Design review of the part shown in the three views and the two pictorial views. Dimensions are in mm from the part's minimum x, y and z. A direction names the side the tool comes from. Give positions to 0.01 mm unless a question says otherwise; leave off trailing zeros. Loops run counter-clockwise (first coordinate to the right, second up) from the corner with the lowest first, then second, coordinate; pieces in that order, holes last. Notation, with made-up numbers: (29, 73) -> (75, 73) arc R17 ccw to (75, 93) -> close; hole circle Ø8 at (4.5, -15). An arc over 180 degrees is marked (long way). Use CSV: the item, a comma, the result in double quotes. Start each with the question number.
Item 1: Clearance check with flat-ended pins moving along their axes: pin 1 (1.6 mm diameter, centred on x = 29.5, y = 1, fed in from -Z); pin 2 (2.5 mm diameter, centred on x = 2.5, z = 33.5, fed in from -Y); pin 3 (1.8 mm diameter, centred on x = 19.5, z = 1.5, fed in from +Y); pin 4 (4 mm diameter, centred on y = 7.5, z = 6.5, fed in from -X). State where each tip first meets the part, or that it passes through.
Item 2: We need section A-A (x = 2.5). State the section outline as (y, z) points.
Item 3: We need section B-B (z = 33.5). State the section outline as (x, y) points.
Item 4: We need section C-C (x = 44.5). State the section outline as (y, z) points.
Item 5: For the marked faces 1, 2 and 3, list the 3-axis set-ups (+Z, -Z, +X, -X, +Y, -Y) from which the entire face can be reached by the end or side of a thin tool; tool diameter is ignored.
Item 6: Wall thickness on line 1 along X through (y, z) = (2.55, 2.5); line 2 along Z through (x, y) = (77.5, 3.1); line 3 along Z through (x, y) = (19, 4.25): over which ranges is each line inside the solid? List them lowest first. Write a range as from..to.
Item 7: We need section D-D (z = 9). State the section outline as (x, y) points.
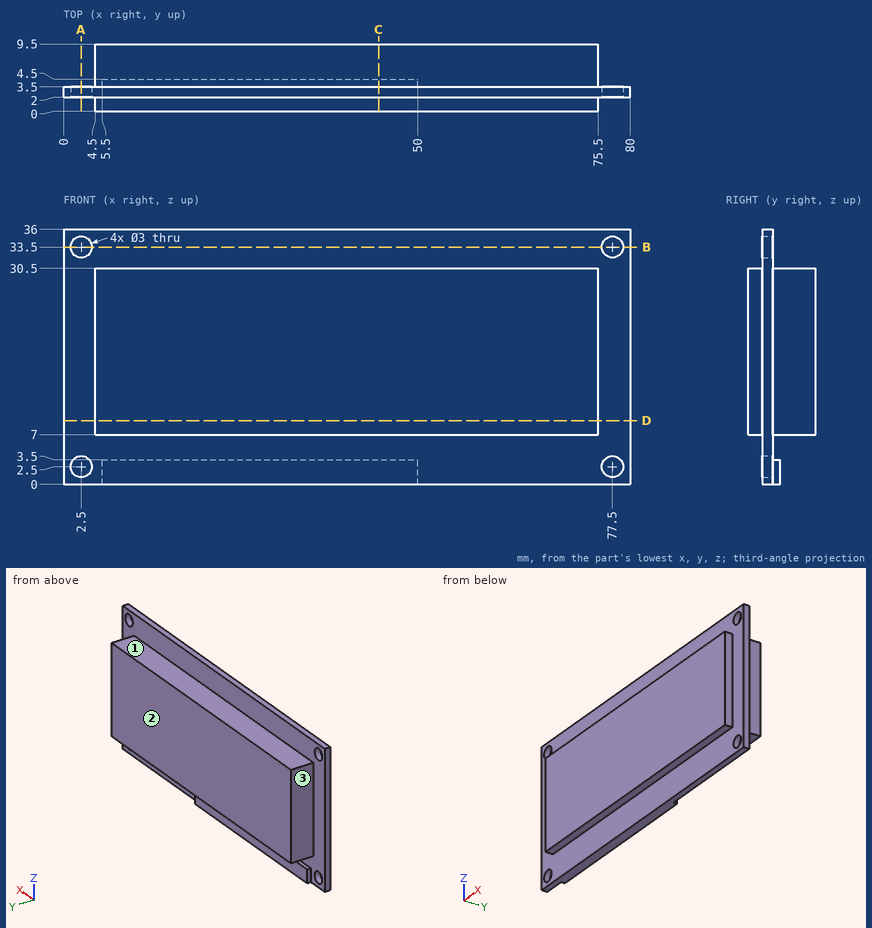
Results found:
1,pin 1,"z = 7"
1,pin 2,"through"
1,pin 3,"y = 4.5"
1,pin 4,"x = 4.5"
2,outline,"(2, 0) -> (3.5, 0) -> (3.5, 1) -> (2, 1) -> close; (2, 4) -> (3.5, 4) -> (3.5, 32) -> (2, 32) -> close; (2, 35) -> (3.5, 35) -> (3.5, 36) -> (2, 36) -> close"
3,outline,"(0, 2) -> (1, 2) -> (1, 3.5) -> (0, 3.5) -> close; (4, 2) -> (76, 2) -> (76, 3.5) -> (4, 3.5) -> close; (79, 2) -> (80, 2) -> (80, 3.5) -> (79, 3.5) -> close"
4,outline,"(0, 7) -> (2, 7) -> (2, 0) -> (4.5, 0) -> (4.5, 3.5) -> (3.5, 3.5) -> (3.5, 7) -> (9.5, 7) -> (9.5, 30.5) -> (3.5, 30.5) -> (3.5, 36) -> (2, 36) -> (2, 30.5) -> (0, 30.5) -> close"
5,face 1,"+Z, +X, -X, +Y"
5,face 2,"+Z, -Z, +X, -X, +Y"
5,face 3,"+Z, -Z, -X, +Y"
6,line 1,"0..1, 4..76, 79..80"
6,line 2,"0..1, 4..32, 35..36"
6,line 3,"0..3.5, 7..30.5"
7,outline,"(0, 2) -> (4.5, 2) -> (4.5, 0) -> (75.5, 0) -> (75.5, 2) -> (80, 2) -> (80, 3.5) -> (75.5, 3.5) -> (75.5, 9.5) -> (4.5, 9.5) -> (4.5, 3.5) -> (0, 3.5) -> close"
